Can you work these out from the model? Positions are in its coordinate system, mm. Coordinates: 2 decimals unless noted, no trailing zeros. Write each loop counter-clockwise with the first axis right and the second up, starting at its lowest first coordinate (ties: lowest second). Pieces come first, ordered by that corner, then holes. Notation, with made-up numbers: (69, 19) -> (101, 19) arc R24 cw to (101, 46) -> close; hole circle Ø3 at (53.5, 50). An arc over 180 degrees is marked (long way). Use one line per item in the form item = value.
```python
from build123d import *

# Parameters (mm, degrees)
F0_R     = 13.7215429526
F1_DEPTH = 7


# Not quite as in the source:
# - a feature names something its author has since deleted; it is built from what else it names


with BuildPart() as f1:
    # F0 (on Top) → F1 (new body)
    with BuildSketch(Plane.XY):
        with BuildLine():
            ThreePointArc((14.9110873094, 6.3741742194), (15.8866974997, 3.2532236753), (16.216368944, 0))
            ThreePointArc((16.216368944, 0), (16.1945778873, -0.8403979891), (16.1292632815, -1.6785373763))
            ThreePointArc((16.1292632815, -1.6785373763), (20.8333456957, -1.1898932874), (25.3830228197, -2.4812501212))
            ThreePointArc((25.3830228197, -2.4812501212), (35.6967714149, -8.0901996637), (42.370743035, 1.5685698162))
            ThreePointArc((42.370743035, 1.5685698162), (35.2903205619, 20.8670320083), (19.9436064757, 34.5433397021))
            ThreePointArc((19.9436064757, 34.5433397021), (24.6328655558, 21.9854776837), (23.6756761013, 8.6148816783))
            ThreePointArc((23.6756761013, 8.6148816783), (19.495827516, 6.702655598), (14.9110873094, 6.3741742194))
        make_face()
        Polygon((35.2634771892, 10.4077201887), (40.3816163825, 4.9971147515), (38.2549642206, -2.1406265287), (31.0101728654, -3.8677623716), (25.8920336721, 1.5428430657), (28.018685834, 8.6805843458), align=None, mode=Mode.SUBTRACT)
        with BuildLine():
            ThreePointArc((16.1292632815, -1.6785373763), (16.1945778873, -0.8403979891), (16.216368944, 0))
            ThreePointArc((16.216368944, 0), (15.8866974997, 3.2532236753), (14.9110873094, 6.3741742194))
            ThreePointArc((14.9110873094, 6.3741742194), (5.9163939381, 15.0985729292), (-6.6109756317, 14.8076204343))
            ThreePointArc((-6.6109756317, 14.8076204343), (-10.1175507485, 12.6730339138), (-12.9757404569, 9.7262932983))
            ThreePointArc((-12.9757404569, 9.7262932983), (-16.0339446866, -2.4255390154), (-9.5182876499, -13.129083058))
            ThreePointArc((-9.5182876499, -13.129083058), (-5.9163939381, -15.0985729292), (-1.9353468525, -16.1004675177))
            ThreePointArc((-1.9353468525, -16.1004675177), (10.1175507485, -12.6730339138), (16.1292632815, -1.6785373763))
        make_face()
        Circle(F0_R, mode=Mode.SUBTRACT)
        with BuildLine():
            ThreePointArc((-4.3771316667, -24.8111777947), (-3.9432437373, -20.2352096957), (-1.9353468525, -16.1004675177))
            ThreePointArc((-1.9353468525, -16.1004675177), (-5.9163939381, -15.0985729292), (-9.5182876499, -13.129083058))
            ThreePointArc((-9.5182876499, -13.129083058), (-11.4471506626, -17.4472599746), (-14.840337048, -20.7417175261))
            ThreePointArc((-14.840337048, -20.7417175261), (-24.8547041379, -26.8692110465), (-19.826950209, -37.4784247537))
            ThreePointArc((-19.826950209, -37.4784247537), (0.4262195398, -40.9958301185), (19.9436064757, -34.5433397021))
            ThreePointArc((19.9436064757, -34.5433397021), (6.7235494105, -32.3254261812), (-4.3771316667, -24.8111777947))
        make_face()
        Polygon((-8.6183885157, -35.742927166), (-15.8631798709, -37.4700630089), (-20.9813190642, -32.0594575716), (-18.8546669023, -24.9217162914), (-11.6098755471, -23.1945804485), (-6.4917363538, -28.6051858858), align=None, mode=Mode.SUBTRACT)
        with BuildLine():
            ThreePointArc((-12.9757404569, 9.7262932983), (-10.1175507485, 12.6730339138), (-6.6109756317, 14.8076204343))
            ThreePointArc((-6.6109756317, 14.8076204343), (-9.3861950332, 18.637153262), (-10.5426857718, 23.2229676473))
            ThreePointArc((-10.5426857718, 23.2229676473), (-10.8420672769, 34.9594107102), (-22.543792826, 35.9098549374))
            ThreePointArc((-22.543792826, 35.9098549374), (-35.7165401018, 20.1287981101), (-39.8872129515, 0))
            ThreePointArc((-39.8872129515, 0), (-31.3564149663, 10.3399484975), (-19.2985444346, 16.1962961164))
            ThreePointArc((-19.2985444346, 16.1962961164), (-15.5525837787, 13.5325540977), (-12.9757404569, 9.7262932983))
        make_face()
        Polygon((-24.5184365116, 32.4729482574), (-17.2736451565, 34.2000841003), (-12.1555059631, 28.789478663), (-14.282158125, 21.6517373829), (-21.5269494802, 19.92460154), (-26.6450886735, 25.3352069772), align=None, mode=Mode.SUBTRACT)
    extrude(amount=F1_DEPTH)


solid = f1.part
```
Q1. Thinking about a two-plate mould opening in Y: for faces 1 (the cylindrical face through (-24.802, -26.697, 3.451)), 2 (the flat face through (-14, -2, 0)), 3 (the cylindrical face through (0.136, -41.016, 3.451)), 4 (the flat face through (-13.204, 25.271, 3.451)), which applies, released by +Y, released by -Y, zero draft, split by the parting line, or undercut?
Return value:
face_1 = undercut
face_2 = zero draft
face_3 = released by -Y
face_4 = undercut
Q2. Will these pins go through, and if not, where does the flat tip stop? pin 1 (2 mm diameter, centred on x = -31.5, z = 3.5, fed in from -Y); pin 2 (2 mm diameter, centred on x = -25, z = 6, fed in from +Y); pin 3 (4 mm diameter, centred on y = -9.5, z = 2.5, fed in from +X).
Return value:
pin_1 = 9.4
pin_2 = 34.8
pin_3 = 37.39
Q3. If I drill on line 1 (X direction, y = 27, z = 5.5); line 2 (Y direction, x = 0, z = 4.5); line 3 (X direction, y = 14.5, z = 5.5), over which ranges is the centre line in solid material (lowest first)? Write a range as from..to.
Return value:
line_1 = -31.55..-26.15, -12.69..-8.65, 23.49..30.21
line_2 = -41.03..-28.63, -16.22..-13.72, 13.72..16.22
line_3 = -37.95..-24.37, -16.61..7.26, 24.81..38.86
Q4. Suppose I cut it at A-A (y = -26). Write out the boundary of the cut face in (x, z), then the cut area to 3 significant figures.
Return value:
outline = (-24.55, 0) -> (-19.18, 0) -> (-19.18, 7) -> (-24.55, 7) -> close; (-8.96, 0) -> (-3.18, 0) -> (-3.18, 7) -> (-8.96, 7) -> close
area = 78.0 mm2
Q5. Suppose I cut it at B-B (y = 4). Write out the boundary of the cut face in (x, z), then the cut area to 3 significant figures.
Return value:
outline = (-39.86, 0) -> (-37.44, 0) -> (-37.44, 7) -> (-39.86, 7) -> close; (-15.72, 0) -> (-13.13, 0) -> (-13.13, 7) -> (-15.72, 7) -> close; (13.13, 0) -> (26.62, 0) -> (26.62, 7) -> (13.13, 7) -> close; (40.08, 0) -> (42.04, 0) -> (42.04, 7) -> (40.08, 7) -> close
area = 143 mm2
Q6. Suppose I cut it at C-C (x = 0). Write out the boundary of the cut face in (y, z), then the cut area to 3 significant figures.
Return value:
outline = (-41.03, 0) -> (-28.63, 0) -> (-28.63, 7) -> (-41.03, 7) -> close; (-16.22, 0) -> (-13.72, 0) -> (-13.72, 7) -> (-16.22, 7) -> close; (13.72, 0) -> (16.22, 0) -> (16.22, 7) -> (13.72, 7) -> close
area = 122 mm2
Q7. Suppose I cut it at D-D (y = -6.5). Write out the boundary of the cut face in (x, z).
Return value:
outline = (-14.86, 0) -> (-12.08, 0) -> (-12.08, 7) -> (-14.86, 7) -> close; (12.08, 0) -> (14.86, 0) -> (14.86, 7) -> (12.08, 7) -> close; (28.3, 0) -> (39.03, 0) -> (39.03, 7) -> (28.3, 7) -> close
